Geometry check sheet. Reference: the model listing, model coordinates, mm. A direction names the side the tool comes from. Coordinates: 2 decimals unless noted, no trailing zeros. Order: outer loops, then holes, each group sorted by start corner. A loop starts at its lowest first (then second) coordinate and runs counter-clockwise, first axis right, second up. Notation, with made-up numbers: (26, 38) - (39, 38) arc R15 ccw to (39, 45) - close; hole circle Ø11 at (28, 46). An arc over 180 degrees is marked (long way). Put each result on its own line as item: value.
from build123d import *

# Parameters (mm, degrees)
F1_DEPTH = 6.985
F2_R     = 50.8
F3_R     = 0.762
F4_R     = 0.762


with BuildPart() as f1:
    # F0 (on Top) → F1 (new body)
    with BuildSketch(Plane.XY):
        with BuildLine():
            ThreePointArc((-6.2554756572, 15.9630839534), (-3.1830763908, 16.8469299782), (0, 17.145))
            ThreePointArc((0, 17.145), (3.1830763908, 16.8469299782), (6.2554756572, 15.9630839534))
            ThreePointArc((6.2554756572, 15.9630839534), (9.5294349524, 17.8680335914), (12.2562140059, 20.4971624553))
            ThreePointArc((12.2562140059, 20.4971624553), (14.8931175874, 25.1821819838), (15.8073346015, 30.48))
            ThreePointArc((15.8073346015, 30.48), (0, 46.2873346015), (-15.8073346015, 30.48))
            ThreePointArc((-15.8073346015, 30.48), (-14.8931175874, 25.1821819838), (-12.2562140059, 20.4971624553))
            ThreePointArc((-12.2562140059, 20.4971624553), (-9.5294349524, 17.8680335914), (-6.2554756572, 15.9630839534))
        make_face()
        with BuildLine():
            ThreePointArc((11.0109, 30.48), (7.785882057, 22.694117943), (0, 19.4691))
            ThreePointArc((0, 19.4691), (-7.785882057, 38.265882057), (11.0109, 30.48))
        make_face(mode=Mode.SUBTRACT)
        with BuildLine():
            ThreePointArc((16.952174055, -2.5641411448), (16.1814075323, -5.6668399724), (14.8480055479, -8.5725))
            ThreePointArc((14.8480055479, -8.5725), (12.9983311415, -11.1800900057), (10.6966983977, -13.3989428086))
            ThreePointArc((10.6966983977, -13.3989428086), (10.6705675574, -16.8425957477), (11.3908194918, -20.2101862123))
            ThreePointArc((11.3908194918, -20.2101862123), (13.5737626184, -24.4839388278), (16.9385483902, -27.9056955145))
            ThreePointArc((16.9385483902, -27.9056955145), (33.4805048345, -29.3711024104), (42.2037889088, -15.24))
            ThreePointArc((42.2037889088, -15.24), (38.9705171928, -5.6606070257), (30.5933849958, 0))
            ThreePointArc((30.5933849958, 0), (26.3964543073, 0.5673346015), (22.1995236189, 0))
            ThreePointArc((22.1995236189, 0), (19.456399269, -1.0376247315), (16.952174055, -2.5641411448))
        make_face()
        with BuildLine():
            ThreePointArc((37.4073543073, -15.24), (23.5466236836, -25.8757126807), (16.8607351888, -9.73455))
            ThreePointArc((16.8607351888, -9.73455), (29.2462849311, -4.6042873193), (37.4073543073, -15.24))
        make_face(mode=Mode.SUBTRACT)
        with BuildLine():
            ThreePointArc((-10.6966983977, -13.3989428086), (-12.9983311415, -11.1800900057), (-14.8480055479, -8.5725))
            ThreePointArc((-14.8480055479, -8.5725), (-16.1814075323, -5.6668399724), (-16.952174055, -2.5641411448))
            ThreePointArc((-16.952174055, -2.5641411448), (-19.456399269, -1.0376247315), (-22.1995236189, 0))
            ThreePointArc((-22.1995236189, 0), (-26.3964543073, 0.5673346015), (-30.5933849958, 0))
            ThreePointArc((-30.5933849958, 0), (-40.5950959898, -22.1876903772), (-16.9385483902, -27.9056955145))
            ThreePointArc((-16.9385483902, -27.9056955145), (-13.5737626184, -24.4839388278), (-11.3908194918, -20.2101862123))
            ThreePointArc((-11.3908194918, -20.2101862123), (-10.7908316405, -17.7572144094), (-10.5891197059, -15.24))
            ThreePointArc((-10.5891197059, -15.24), (-10.6160372972, -14.3179012042), (-10.6966983977, -13.3989428086))
        make_face()
        with BuildLine():
            ThreePointArc((-15.3855543073, -15.24), (-37.032166988, -18.0898306237), (-16.8607351888, -9.73455))
            ThreePointArc((-16.8607351888, -9.73455), (-15.7607416267, -12.3901693763), (-15.3855543073, -15.24))
        make_face(mode=Mode.SUBTRACT)
        with BuildLine():
            Line((-22.1995236189, 0), (-12.2562140059, 20.4971624553))
            ThreePointArc((-12.2562140059, 20.4971624553), (-14.8931175874, 25.1821819838), (-15.8073346015, 30.48))
            Line((-15.8073346015, 30.48), (-30.5933849958, 0))
            ThreePointArc((-30.5933849958, 0), (-26.3964543073, 0.5673346015), (-22.1995236189, 0))
        make_face()
        with BuildLine():
            ThreePointArc((15.8073346015, 30.48), (14.8931175874, 25.1821819838), (12.2562140059, 20.4971624553))
            Line((12.2562140059, 20.4971624553), (22.1995236189, 0))
            ThreePointArc((22.1995236189, 0), (26.3964543073, 0.5673346015), (30.5933849958, 0))
            Line((30.5933849958, 0), (15.8073346015, 30.48))
        make_face()
        with BuildLine():
            ThreePointArc((16.9385483902, -27.9056955145), (13.5737626184, -24.4839388278), (11.3908194918, -20.2101862123))
            Line((11.3908194918, -20.2101862123), (-11.3908194918, -20.2101862123))
            ThreePointArc((-11.3908194918, -20.2101862123), (-13.5737626184, -24.4839388278), (-16.9385483902, -27.9056955145))
            Line((-16.9385483902, -27.9056955145), (16.9385483902, -27.9056955145))
        make_face()
        with BuildLine():
            ThreePointArc((0, 11.0109), (7.785882057, 7.785882057), (11.0109, 0))
            ThreePointArc((11.0109, 0), (10.6357126807, -2.8498306237), (9.5357191185, -5.50545))
            Line((9.5357191185, -5.50545), (12.7069009763, -7.3363326993))
            ThreePointArc((12.7069009763, -7.3363326993), (14.5859921181, -4.7335824336), (16.952174055, -2.5641411448))
            ThreePointArc((16.952174055, -2.5641411448), (17.0967255516, -1.2856906369), (17.145, 0))
            ThreePointArc((17.145, 0), (14.1633533307, 9.6618035288), (6.2554756572, 15.9630839534))
            ThreePointArc((6.2554756572, 15.9630839534), (3.1935934206, 14.9986309305), (0, 14.6726653985))
            Line((0, 14.6726653985), (0, 11.0109))
        make_face()
        with BuildLine():
            Line((12.7069009763, -7.3363326993), (9.5357191185, -5.50545))
            ThreePointArc((9.5357191185, -5.50545), (0, -11.0109), (-9.5357191185, -5.50545))
            Line((-9.5357191185, -5.50545), (-12.7069009763, -7.3363326993))
            ThreePointArc((-12.7069009763, -7.3363326993), (-11.3923986975, -10.2650484968), (-10.6966983977, -13.3989428086))
            ThreePointArc((-10.6966983977, -13.3989428086), (0, -17.145), (10.6966983977, -13.3989428086))
            ThreePointArc((10.6966983977, -13.3989428086), (11.3923986975, -10.2650484968), (12.7069009763, -7.3363326993))
        make_face()
        with BuildLine():
            ThreePointArc((-9.5357191185, -5.50545), (-9.5357191185, 5.50545), (0, 11.0109))
            Line((0, 11.0109), (0, 14.6726653985))
            ThreePointArc((0, 14.6726653985), (-3.1935934206, 14.9986309305), (-6.2554756572, 15.9630839534))
            ThreePointArc((-6.2554756572, 15.9630839534), (-14.8480055479, 8.5725), (-16.952174055, -2.5641411448))
            ThreePointArc((-16.952174055, -2.5641411448), (-14.5859921181, -4.7335824336), (-12.7069009763, -7.3363326993))
            Line((-12.7069009763, -7.3363326993), (-9.5357191185, -5.50545))
        make_face()
        with BuildLine():
            Line((14.8480055479, -8.5725), (12.7069009763, -7.3363326993))
            ThreePointArc((12.7069009763, -7.3363326993), (11.3923986975, -10.2650484968), (10.6966983977, -13.3989428086))
            ThreePointArc((10.6966983977, -13.3989428086), (12.9983311415, -11.1800900057), (14.8480055479, -8.5725))
        make_face()
        with BuildLine():
            ThreePointArc((16.952174055, -2.5641411448), (14.5859921181, -4.7335824336), (12.7069009763, -7.3363326993))
            Line((12.7069009763, -7.3363326993), (14.8480055479, -8.5725))
            ThreePointArc((14.8480055479, -8.5725), (16.1814075323, -5.6668399724), (16.952174055, -2.5641411448))
        make_face()
        with BuildLine():
            Line((0, 17.145), (0, 14.6726653985))
            ThreePointArc((0, 14.6726653985), (3.1935934206, 14.9986309305), (6.2554756572, 15.9630839534))
            ThreePointArc((6.2554756572, 15.9630839534), (3.1830763908, 16.8469299782), (0, 17.145))
        make_face()
        with BuildLine():
            ThreePointArc((-6.2554756572, 15.9630839534), (-3.1935934206, 14.9986309305), (0, 14.6726653985))
            Line((0, 14.6726653985), (0, 17.145))
            ThreePointArc((0, 17.145), (-3.1830763908, 16.8469299782), (-6.2554756572, 15.9630839534))
        make_face()
        with BuildLine():
            Line((-14.8480055479, -8.5725), (-12.7069009763, -7.3363326993))
            ThreePointArc((-12.7069009763, -7.3363326993), (-14.5859921181, -4.7335824336), (-16.952174055, -2.5641411448))
            ThreePointArc((-16.952174055, -2.5641411448), (-16.1814075323, -5.6668399724), (-14.8480055479, -8.5725))
        make_face()
        with BuildLine():
            ThreePointArc((-10.6966983977, -13.3989428086), (-11.3923986975, -10.2650484968), (-12.7069009763, -7.3363326993))
            Line((-12.7069009763, -7.3363326993), (-14.8480055479, -8.5725))
            ThreePointArc((-14.8480055479, -8.5725), (-12.9983311415, -11.1800900057), (-10.6966983977, -13.3989428086))
        make_face()
    extrude(amount=F1_DEPTH)

    # F2
    f2_edges = [f1.edges().sort_by_distance(p)[0] for p in [
        (16.938548, -27.905696, 3.4925),
        (-16.938548, -27.905696, 3.4925),
        (15.807335, 30.48, 3.4925),
        (30.593385, 0, 3.4925),
        (-15.807335, 30.48, 3.4925),
        (-30.593385, 0, 3.4925),
    ]]
    fillet(f2_edges, radius=F2_R)

    # F3
    f3_edges = [f1.edges().sort_by_distance(p)[0] for p in [
        (0, -27.905696, 0),
    ]]
    fillet(f3_edges, radius=F3_R)

    # F4
    f4_edges = [f1.edges().sort_by_distance(p)[0] for p in [
        (-21.716674, 18.298473, 6.985),
    ]]
    fillet(f4_edges, radius=F4_R)


solid = f1.part
Q1. Thickness scan on L1, parallel to X at y = 8.5, z = 1.5; L2, parallel to X at y = 4, z = 5.75; L3, parallel to Y at x = -18.5, z = 4. Record the ranges inside material, lowest first. Write a range as [from, to].
Answer block:
L1: x = [-26.75, -18.08], [-14.89, -7], [7, 14.89], [18.08, 26.75]
L2: x = [-29.85, -20.26], [-16.67, -10.26], [10.26, 16.67], [20.26, 29.85]
L3: y = [-29.42, -22.91], [-7.57, -1.55], [7.63, 24.97]
Q2. Depth check by flat-ended pin: pin 1 Ø1.6 at (x, z) = (1.5, 3.5) entering from -Y; pin 2 Ø1 at (y, z) = (10.5, 6) entering from +X; pin 3 Ø2 at (y, z) = (14, 5.5) entering from +X. Enter the tip coordinate at first touch or a pass-through.
Answer block:
pin 1: stops at y = -27.91
pin 2: stops at x = 25.86
pin 3: stops at x = 24.29
Q3. Section check A-A on z = 3.75. Record the boundary of the cut face in (x, y) (3 decimals).
Answer block:
outline: (-36.754, -3.298) arc R15.807 ccw to (-21.599, -30.302) arc R50.8 cw to (-6.182, -27.906) - (6.182, -27.906) arc R50.8 cw to (21.599, -30.302) arc R15.807 ccw to (36.754, -3.298) arc R50.8 cw to (24.333, 12.906) - (19.101, 23.691) arc R50.8 cw to (15.38, 34.131) arc R15.807 ccw to (-15.38, 34.131) arc R50.8 cw to (-19.101, 23.691) - (-24.333, 12.906) arc R50.8 cw to start; hole circle Ø22.022 at (-26.396, -15.24); hole (-22.2, 0) arc R15.807 cw to (-16.952, -2.564) arc R17.145 cw to (-6.255, 15.963) arc R15.807 cw to (-12.256, 20.497) - close; hole (-11.391, -20.21) - (11.391, -20.21) arc R15.807 cw to (10.697, -13.399) arc R17.145 cw to (-10.697, -13.399) arc R15.807 cw to start; hole circle Ø22.022 at (0, 0); hole circle Ø22.022 at (0, 30.48); hole (6.255, 15.963) arc R17.145 cw to (16.952, -2.564) arc R15.807 cw to (22.2, 0) - (12.256, 20.497) arc R15.807 cw to start; hole circle Ø22.022 at (26.396, -15.24)
Q4. Section check B-B on x = 2.5. State how many separate pieces and enclosed holes the cut face has, then the cut area to 3 significant figures.
Answer block:
separate pieces: 4
enclosed holes: 0
area: 194 mm^2
Q5. Draft check along Y on faces 1 (the cylindrical face through (9.49, 17.84, 3.44)), 2 (the cylindrical face through (0.296, 46.285, 3.454)), 3 (the cylindrical face through (-40.327, -22.711, 3.454)). Enter one of: pulls with the +Y half, pulls with the -Y half, needs draft (parallel to the pull), parting line crosses it, or undercut.
Answer block:
face 1: undercut
face 2: pulls with the +Y half
face 3: parting line crosses it
Q6. Access from +Z, -Z, +X, -X, +Y, -Y to the whole of each face (thin tool, end or side, straight path). Record for faces 4 (the flat face through (-17.3, 10.1, 3.4)), 5 (the flat face through (21.753, 18.223, 3.454)), 6 (the cylindrical face through (14.091, -28.525, 3.531)).
Answer block:
face 4: +Z, -Z
face 5: +Z, -Z, +X, +Y
face 6: +Z, -Z, -Y
